```python
from build123d import *

# Parameters (mm, degrees)
EXTRUDE_1_DEPTH = 217
FILLET_1_R      = 20


with BuildPart() as part:
    # Эскиз1 → Бобышка-Вытянуть1 (new, symmetric)
    with BuildSketch(Plane.XY):
        Polygon((0, 0), (60, 0), (60, 6), (6, 6), (6, 60), (0, 60), align=None)
    extrude(amount=EXTRUDE_1_DEPTH, both=True)

    # Скругление1
    fillet_1_edges = [part.edges().sort_by_distance(p)[0] for p in [
        (60, 3, 217),
        (3, 60, 217),
        (3, 60, -217),
        (60, 3, -217),
    ]]
    fillet(fillet_1_edges, radius=FILLET_1_R)


solid = part.part
```
Verification items for the finished model (mm, model axes). A direction names the side the tool comes from. Give positions to 0.01 mm unless a question says otherwise; leave off trailing zeros. Loops run counter-clockwise (first coordinate to the right, second up) from the corner with the lowest first, then second, coordinate; pieces in that order, holes last.
1. Section check A-A, the plane y = 20. Enter the section's corners in (x, z).
2. Go/stop test with flat-tipped pins: pin 1 Ø1.5 at (x, z) = (35.5, 105.5) entering from +Y; pin 2 Ø1 at (y, z) = (8.5, 38.5) entering from +X. Record where each tip stops, or that it passes through.
3. Thickness scan on line 1 (Y direction, x = 49.5, z = -66). Record the ranges inside material, lowest first.
4. Section check B-B, the plane z = -163. Enter the section's corners in (x, y).
5. Set-up check for faces 1 (the flat face through (6, 33, 3)), 2 (the cylindrical face through (2.958, 54.297, 210.986)): record each of +Z, -Z, +X, -X, +Y, -Y from which the full face is reachable in a straight line by a thin tool's end or side.
Geometry says:
1. outline: (0, -217) - (6, -217) - (6, 217) - (0, 217) - close
2. pin 1: stops at y = 6
2. pin 2: stops at x = 6
3. line 1: y = 0 to 6
4. outline: (0, 0) - (60, 0) - (60, 6) - (6, 6) - (6, 60) - (0, 60) - close
5. face 1: +Z, -Z, +X, +Y
5. face 2: +Z, +X, -X, +Y
